Could you check a few things on this drawing? It's one solid part, dimensions in mm from its lowest x, y, z. A direction names the side the tool comes from. Round coordinates to 2 decimals unless told otherwise and drop trailing zeros. Write each loop counter-clockwise with the first axis right and the second up, starting at its lowest first coordinate (ties: lowest second). Pieces come first, ordered by that corner, then holes. Notation, with made-up numbers: (60, 19) -> (114, 19) arc R20 cw to (114, 49) -> close; hole circle Ø1 at (-11.75, 59.25). An arc over 180 degrees is marked (long way). Answer in a Markdown table with one row per item.
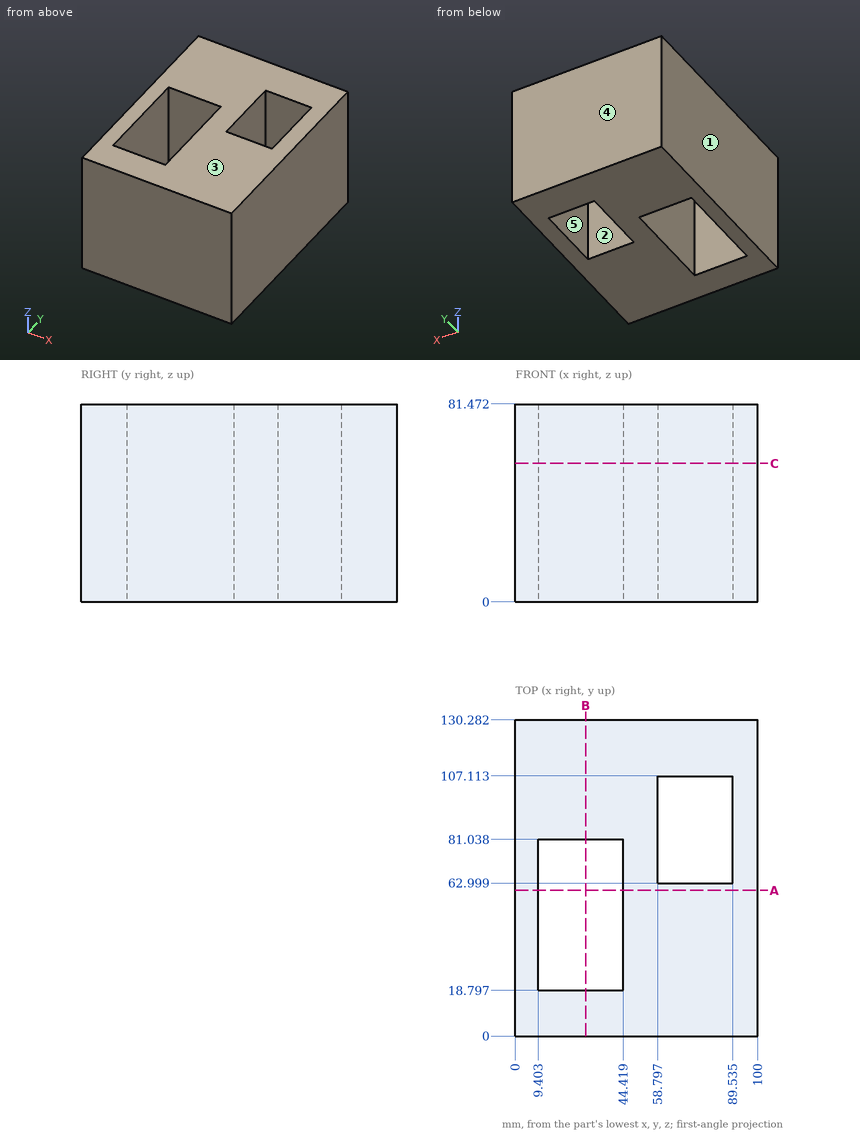
1) I want a section at C-C, the plane z = 57. List the corners of the cut face in (x, y) for me (1 decimal).
Response:
| item | result |
|---|---|
| outline | (0, 0) -> (100, 0) -> (100, 130.3) -> (0, 130.3) -> close; hole (9.4, 18.8) -> (44.4, 18.8) -> (44.4, 81) -> (9.4, 81) -> close; hole (58.8, 63) -> (89.5, 63) -> (89.5, 107.1) -> (58.8, 107.1) -> close |
2) I want a section at A-A, the plane y = 60. List the corners of the cut face in (x, z) for me.
Response:
| item | result |
|---|---|
| outline | (0, 0) -> (9.4, 0) -> (9.4, 81.47) -> (0, 81.47) -> close; (44.42, 0) -> (100, 0) -> (100, 81.47) -> (44.42, 81.47) -> close |
3) Which directions (+Z, -Z, +X, -X, +Y, -Y) give clear straight access to the entire face, cutting with the end or side of a thin tool? Please do the marked faces 1 and 2.
Response:
| item | result |
|---|---|
| face 1 | +Z, -Z, -X, +Y, -Y |
| face 2 | +Z, -Z |
4) We'd pull the mould along Y, two halves only. Please class the marked faces 3, 4 and 5: +Y half, -Y half, draft (parallel to the pull), parting line (faces both ways), or undercut.
Response:
| item | result |
|---|---|
| face 3 | draft |
| face 4 | +Y half |
| face 5 | undercut |
5) I want a section at B-B, the plane x = 29. List the corners of the cut face in (y, z) for me.
Response:
| item | result |
|---|---|
| outline | (0, 0) -> (18.8, 0) -> (18.8, 81.47) -> (0, 81.47) -> close; (81.04, 0) -> (130.28, 0) -> (130.28, 81.47) -> (81.04, 81.47) -> close |
6) I need wall thicknesses on line 1 (X direction, y = 67, z = 63.5) (1 decimal); line 2 (X direction, y = 48, z = 54); line 3 (Y direction, x = 66, z = 7). Which ranges of each line are inside material? Lowest first, please. Write a range as [from, to].
Response:
| item | result |
|---|---|
| line 1 | x = [0, 9.4], [44.4, 58.8], [89.5, 100] |
| line 2 | x = [0, 9.4], [44.42, 100] |
| line 3 | y = [0, 63], [107.11, 130.28] |
